Design review of the part built by this model. Coordinates are the model's own, in mm. Face numbers are marked on the shaded views. A direction names the side the tool comes from. Round coordinates to 2 decimals unless told otherwise and drop trailing zeros. Loops run counter-clockwise (first coordinate to the right, second up) from the corner with the lowest first, then second, coordinate; pieces in that order, holes last. Notation, with made-up numbers: (61.25, -6.5) -> (98.25, -6.5) arc R20 ccw to (98.25, 29.5) -> close; hole circle Ø10 at (27, 77.25). An arc over 180 degrees is marked (long way). Answer as CSV lines item,"result". Start each with the question number.
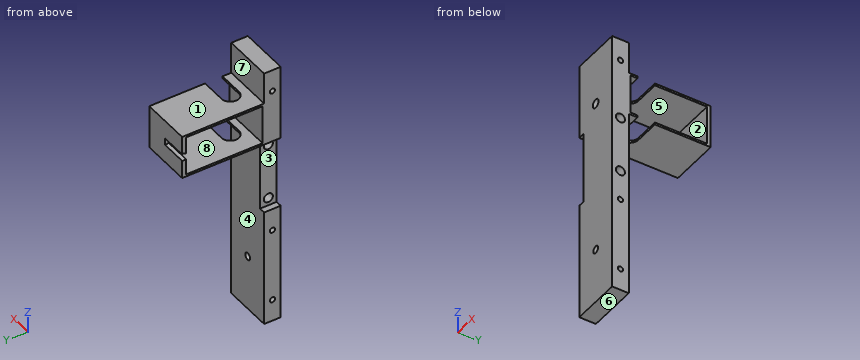
```python
from build123d import *

# Parameters (mm, degrees)
SKETCH2_W             = 28.575
SKETCH2_H             = 152.4
BOSS_EXTRUDE1_DEPTH   = 9.525
F_3_0MM_DOWEL_HOLE1_D = 3
LPATTERN1_COUNT       = 4
LPATTERN1_PITCH       = 42.333333333
SKETCH12_R            = 2.05
CUT_EXTRUDE1_DEPTH    = 156.348048749
SKETCH12_4_R          = 10.975
CUT_EXTRUDE2_DEPTH    = 4
SKETCH15_R            = 2.5
CUT_EXTRUDE3_DEPTH    = 156.154169296
SKETCH13_R            = 2.6
CUT_EXTRUDE4_DEPTH    = 156.348048749
SKETCH17_W            = 41.28
SKETCH17_H            = 9.525
CUT_EXTRUDE5_DEPTH    = 3.575
SKETCH18_W            = 28.575
SKETCH18_H            = 25
BOSS_EXTRUDE3_DEPTH   = 47
CUT_EXTRUDE12_REACH   = 167.037
SKETCH19_W            = 22.5
SKETCH19_H            = 44
CUT_EXTRUDE18_DEPTH   = 15
CUT_EXTRUDE17_DEPTH   = 25


with BuildPart() as part:
    # Sketch2 → Boss-Extrude1 (new body)
    with BuildSketch(Plane(origin=(0, 0, 0), x_dir=(1, 0, 0), z_dir=(0, 1, 0))):
        with Locations((14.2875, 76.2)):
            Rectangle(SKETCH2_W, SKETCH2_H)
    extrude(amount=BOSS_EXTRUDE1_DEPTH)

    # Ø3.0mm Dowel Hole1 (through all)
    with Locations(Plane.ZY):
        with Locations((-139.7, 4.7625)):
            f_3_0mm_dowel_hole1 = Hole(F_3_0MM_DOWEL_HOLE1_D / 2)

    # LPattern1: Ø3.0mm Dowel Hole1 ×4, 1 skipped
    with Locations(*[(0, 0, i * LPATTERN1_PITCH) for i in range(1, LPATTERN1_COUNT) if i not in (2,)]):
        add(f_3_0mm_dowel_hole1, mode=Mode.SUBTRACT)

    # Sketch12 → Cut-Extrude1 (cut, through all)
    with BuildSketch(Plane(origin=(0, 9.525, 0), x_dir=(1, 0, 0), z_dir=(0, 1, 0))):
        with Locations(Location((14.2875, 120.65, 0), (0, 0, 270))):
            Circle(SKETCH12_R)
    extrude(amount=-CUT_EXTRUDE1_DEPTH, mode=Mode.SUBTRACT)

    # Sketch12<4> → Cut-Extrude2 (cut)
    with BuildSketch(Plane(origin=(0, 9.525, 0), x_dir=(1, 0, 0), z_dir=(0, 1, 0))):
        with Locations(Location((14.2875, 31.75, 0), (0, 0, 270))):
            Circle(SKETCH12_4_R)
    extrude(amount=-CUT_EXTRUDE2_DEPTH, mode=Mode.SUBTRACT)

    # Sketch15 → Cut-Extrude3 (cut, through all)
    with BuildSketch(Plane(origin=(0, 5.525, 0), x_dir=(1, 0, 0), z_dir=(0, 1, 0))):
        with Locations(Location((14.2875, 31.75, 0), (0, 0, 270))):
            Circle(SKETCH15_R)
    extrude(amount=-CUT_EXTRUDE3_DEPTH, mode=Mode.SUBTRACT)

    # Sketch13 → Cut-Extrude4 (cut, through all)
    with BuildSketch(Plane.ZY):
        with Locations((-80, 4.7625)):
            Circle(SKETCH13_R)
        with Locations((-47.79, 4.7625)):
            Circle(SKETCH13_R)
    extrude(amount=-CUT_EXTRUDE4_DEPTH, mode=Mode.SUBTRACT)

    # Sketch17 → Cut-Extrude5 (cut)
    with BuildSketch(Plane.ZY):
        with Locations((-63.895, 4.7625)):
            Rectangle(SKETCH17_W, SKETCH17_H)
    extrude(amount=-CUT_EXTRUDE5_DEPTH, mode=Mode.SUBTRACT)

    # Sketch18 → Boss-Extrude3 (add)
    with BuildSketch(Plane(origin=(0, 9.525, 0), x_dir=(1, 0, 0), z_dir=(0, 1, 0))):
        with Locations((14.2875, 30.755)):
            Rectangle(SKETCH18_W, SKETCH18_H)
    extrude(amount=BOSS_EXTRUDE3_DEPTH)

    # Sketch19 → Cut-Extrude12 (cut, up to next)
    with BuildSketch(Plane.ZY, mode=Mode.PRIVATE) as cut_extrude12_sk1:
        with Locations((-30.755, 32.413500749)):
            Rectangle(SKETCH19_W, SKETCH19_H)
    cut_extrude12_tool1 = extrude(cut_extrude12_sk1.sketch, amount=-CUT_EXTRUDE12_REACH, mode=Mode.PRIVATE) & part.part
    add(cut_extrude12_tool1.solids().sort_by_distance((0, 32.413501, -30.755))[0], mode=Mode.SUBTRACT)

    # Sketch20 → Cut-Extrude18 (cut)
    with BuildSketch(Plane.ZY):
        with BuildLine():
            Line((-32.81559427, 56.525), (-28.887718849, 56.525))
            ThreePointArc((-28.887718849, 56.525), (-30.851656559, 53.588833805), (-32.81559427, 56.525))
        make_face()
    extrude(amount=-CUT_EXTRUDE18_DEPTH, mode=Mode.SUBTRACT)

    # Sketch21 → Cut-Extrude17 (cut)
    with BuildSketch(Plane.XY.offset(-18.255)):
        with BuildLine():
            Line((14.2875, 24.525), (28.575, 24.525))
            Line((28.575, 24.525), (28.575, 14.525))
            Line((28.575, 14.525), (14.2875, 14.525))
            ThreePointArc((14.2875, 14.525), (9.2875, 19.525), (14.2875, 24.525))
        make_face()
    extrude(amount=-CUT_EXTRUDE17_DEPTH, mode=Mode.SUBTRACT)


solid = part.part
```
Q1. Mouldability with a two-part tool opening along Z and no side actions: class the marked faces 5, 6, 7 and 8 as pulls with the +Z half, pulls with the -Z half, needs draft (parallel to the pull), parting line crosses it, or undercut.
Q2. Machinability: for the marked faces 1, 2, 3 and 4, which of the approach directions +Z, -Z, +X, -X, +Y, -Y give a long, thin tool a straight path to every point of the face, cutting with its end or side? Answer none if there is none.
Q3. Add section A-A, the plane y = 49. Give the boundary of the cut face in (x, z) (3 decimals), and give its area (3 significant figures).
Q4. Add section D-D, the plane x = 26.75. Give the boundary of the cut face in (y, z) (1 decimal), and give its area (3 significant figures).
Q5. To check wall thickness, follow probe 1 along Z at (x, y) = (26, 53.5) (3 decimals); probe 2 along Y at (x, z) = (13.75, -47.79) (1 decimal); probe 3 along Y at (x, z) = (2, -13) (3 decimals). State the ranges of each line that lie inside material, in increasing order. Write a range as from..to.
Q6. Add section B-B, the plane x = 19.25. State how many separate pieces and enclosed holes the cut face has, and give its area (3 significant figures).
Q7. For pin 1 Ø0.6 at (x, z) = (23, -43) entering from -Y; pin 2 Ø5.5 at (x, z) = (15, -12) entering from +Y (3 decimals); pin 3 Ø8.5 at (y, z) = (4.76, -80) entering from -X (3 decimals); pin 4 Ø1.5 at (x, y) = (6, 35) entering from +Z (3 decimals), all flat-tipped, find the tip position at first contact; note any pin that passes through.
Q8. Add section C-C, the plane z = -47.79. Give the boundary of the cut face in (x, y) (1 decimal).
Worked answers:
1,face 5,"undercut"
1,face 6,"pulls with the -Z half"
1,face 7,"needs draft"
1,face 8,"undercut"
2,face 1,"+Z, +X, -X, +Y"
2,face 2,"+X, -X"
2,face 3,"-X, +Y, -Y"
2,face 4,"-Z, +X, -X, +Y"
3,outline,"(0, -43.255) -> (28.575, -43.255) -> (28.575, -42.005) -> (0, -42.005) -> close; (0, -19.505) -> (28.575, -19.505) -> (28.575, -18.255) -> (0, -18.255) -> close"
3,area,"71.4 mm^2"
4,outline,"(0, -152.4) -> (9.5, -152.4) -> (9.5, -43.3) -> (14.5, -43.3) -> (14.5, -42) -> (10.4, -42) -> (10.4, -19.5) -> (14.5, -19.5) -> (14.5, -18.3) -> (9.5, -18.3) -> (9.5, 0) -> (0, 0) -> close; (24.5, -43.3) -> (56.5, -43.3) -> (56.5, -18.3) -> (24.5, -18.3) -> (24.5, -19.5) -> (54.4, -19.5) -> (54.4, -42) -> (24.5, -42) -> close; hole circle Ø5.2 at (4.8, -80); hole circle Ø5.2 at (4.8, -47.8); hole circle Ø3 at (4.8, -139.7); hole circle Ø3 at (4.8, -97.4); hole circle Ø3 at (4.8, -12.7)"
4,area,"1,550 mm^2"
5,probe 1,"z = -43.255..-42.005, -19.505..-18.255"
5,probe 2,"y = 0..2.2, 7.4..9.5"
5,probe 3,"y = 0..3.293, 6.232..9.525"
6,separate pieces,"2"
6,enclosed holes,"6"
6,area,"1,470 mm^2"
7,pin 1,"stops at y = 0"
7,pin 2,"stops at y = 9.525"
7,pin 3,"stops at x = 3.575"
7,pin 4,"stops at z = -18.255"
8,outline,"(3.6, 0) -> (28.6, 0) -> (28.6, 2.2) -> (3.6, 2.2) -> close; (3.6, 7.4) -> (28.6, 7.4) -> (28.6, 9.5) -> (3.6, 9.5) -> close"
